Check sheet for the modelled part. Datum: model origin and axes. Units: mm. Round coordinates to 2 decimals unless told otherwise and drop trailing zeros. Order: outer loops, then holes, each group sorted by start corner. A loop starts at its lowest first (then second) coordinate and runs counter-clockwise, first axis right, second up. Notation, with made-up numbers: (44.25, 24) -> (72.25, 24) arc R29 ccw to (72.25, 53) -> close; hole circle Ø6 at (65.5, 70.5). An arc over 180 degrees is marked (long way). Answer in a Markdown table with one row per item.
```python
from build123d import *

# Parameters (mm, degrees)
F1_DEPTH = 50
F3_D     = 7.9375


with BuildPart() as f1:
    # F0 (on Top) → F1 (new body)
    with BuildSketch(Plane.XY):
        with BuildLine():
            ThreePointArc((0, 9), (9, 0), (0, -9))
            Line((0, -9), (0, -31))
            Line((0, -31), (30, -31))
            Line((30, -31), (30, 29))
            Line((30, 29), (0, 29))
            Line((0, 29), (0, 9))
        make_face()
    extrude(amount=F1_DEPTH)

    # F3 (through all)
    with Locations(Plane.YZ.offset(30)):
        with Locations((-21, 38), (-21, 9.508006103), (18.8892395088, 38), (18.8892395088, 9.508006103)):
            Hole(F3_D / 2)


solid = f1.part
```
(1) Scan lines: probe 1 along Y at (x, z) = (9.75, 40.5); probe 2 along Y at (x, z) = (5.25, 7.5); probe 3 along Y at (x, z) = (25.5, 41). Record each from-to range of solid material in increasing order. Write a range as from..to.
Solutions:
| item | result |
|---|---|
| probe 1 | -31..-24.08, -17.92..15.81, 21.97..29 |
| probe 2 | -31..-24.42, -17.58..-7.31, 7.31..15.47, 22.31..29 |
| probe 3 | -31..-23.6, -18.4..16.29, 21.49..29 |
(2) Draft check along Z on faces 1 (the flat face through (15, -1, 50)), 2 (the cylindrical face through (14.79, -24.666, 36.48)), 3 (the cylindrical face through (9, 0, 25)), 4 (the cylindrical face through (14.79, 22.854, 38.174)). Enter one of: pulls with the +Z half, pulls with the -Z half, needs draft (parallel to the pull), parting line crosses it, or undercut.
Solutions:
| item | result |
|---|---|
| face 1 | pulls with the +Z half |
| face 2 | undercut |
| face 3 | needs draft |
| face 4 | undercut |
(3) Depth check by flat-ended pin: pin 1 Ø5 at (y, z) = (18.89, 38) entering from +X. Enter the tip coordinate at first touch or a pass-through.
Solutions:
| item | result |
|---|---|
| pin 1 | through |
(4) Section check C-C on x = 20. Record the boundary of the cut face in (y, z).
Solutions:
| item | result |
|---|---|
| outline | (-31, 0) -> (29, 0) -> (29, 50) -> (-31, 50) -> close; hole circle Ø7.94 at (-21, 9.51); hole circle Ø7.94 at (-21, 38); hole circle Ø7.94 at (18.89, 9.51); hole circle Ø7.94 at (18.89, 38) |
(5) Section check D-D on z = 15.5. Record the boundary of the cut face in (x, y).
Solutions:
| item | result |
|---|---|
| outline | (0, -31) -> (30, -31) -> (30, 29) -> (0, 29) -> (0, 9) arc R9 cw to (0, -9) -> close |
(6) Section check A-A on y = -21. Record the boundary of the cut face in (x, z).
Solutions:
| item | result |
|---|---|
| outline | (0, 0) -> (30, 0) -> (30, 5.54) -> (0, 5.54) -> close; (0, 13.48) -> (30, 13.48) -> (30, 34.03) -> (0, 34.03) -> close; (0, 41.97) -> (30, 41.97) -> (30, 50) -> (0, 50) -> close |
(7) Section check B-B on z = 38. Record the boundary of the cut face in (x, y).
Solutions:
| item | result |
|---|---|
| outline | (0, -31) -> (30, -31) -> (30, -24.97) -> (0, -24.97) -> close; (0, -17.03) -> (30, -17.03) -> (30, 14.92) -> (0, 14.92) -> (0, 9) arc R9 cw to (0, -9) -> close; (0, 22.86) -> (30, 22.86) -> (30, 29) -> (0, 29) -> close |
